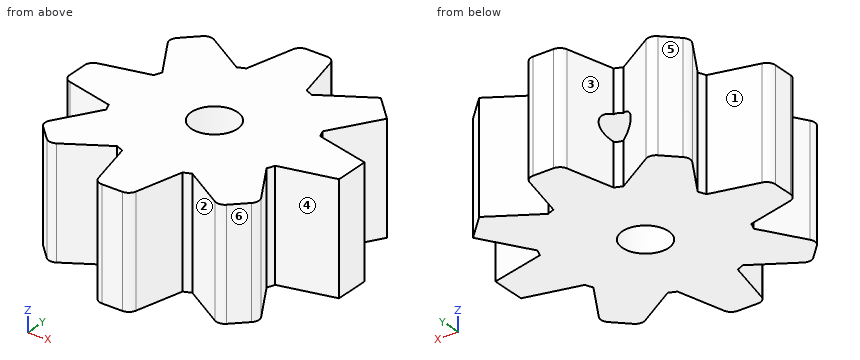
from build123d import *

# Parameters (mm, degrees)
SKETCH1_R                      = 10
SKETCH1_R_2                    = 2.6
BOSS_EXTRUDE1_DEPTH            = 12.4
BOSS_EXTRUDE2_DEPTH            = 6.2
CIRPATTERN1_DEPTH              = 12.4
CUT_EXTRUDE1_REACH             = 35.782
CUT_EXTRUDE1_END_RADIUS        = 2.6
SKETCH5_R                      = 1.5
CUT_EXTRUDE1_DIRECTION_2_DEPTH = 4.1
FILLET4_R                      = 1


# Read off the part's stored shape, not the designer's step: CirPattern1
with BuildPart() as part:
    # Sketch1 → Boss-Extrude1 (new body)
    with BuildSketch(Plane.XY):
        with Locations(Location((0, 0, 0), (0, 0, 180))):
            Circle(SKETCH1_R)
        with Locations(Location((0, 0, 0), (0, 0, 180))):
            Circle(SKETCH1_R_2, mode=Mode.SUBTRACT)
    extrude(amount=BOSS_EXTRUDE1_DEPTH)

    # Sketch2 → Boss-Extrude2 (add, symmetric)
    with BuildSketch(Plane.XY.offset(6.2)):
        Polygon((-1.935099749, 15.52158862), (-3.5, 9), (3.5, 9), (1.935099749, 15.52158862), align=None)
    extrude(amount=BOSS_EXTRUDE2_DEPTH, both=True)

    # CirPattern1 outline → CirPattern1 (add)
    with BuildSketch(Plane.XY):
        with BuildLine():
            Line((-9.607098413, 12.343742723), (-12.343742723, 9.607098413))
            Line((-12.343742723, 9.607098413), (-9.055455951, 4.242489544))
            ThreePointArc((-9.055455951, 4.242489544), (-7.071067812, 7.071067812), (-4.242489544, 9.055455951))
            Line((-4.242489544, 9.055455951), (-9.607098413, 12.343742723))
        make_face()
        with BuildLine():
            ThreePointArc((4.242489544, 9.055455951), (7.071067812, 7.071067812), (9.055455951, 4.242489544))
            Line((9.055455951, 4.242489544), (12.343742723, 9.607098413))
            Line((12.343742723, 9.607098413), (9.607098413, 12.343742723))
            Line((9.607098413, 12.343742723), (4.242489544, 9.055455951))
        make_face()
        with BuildLine():
            ThreePointArc((9.403067435, 3.403281184), (10, 0), (9.403067435, -3.403281184))
            Line((9.403067435, -3.403281184), (15.52158862, -1.935099749))
            Line((15.52158862, -1.935099749), (15.52158862, 1.935099749))
            Line((15.52158862, 1.935099749), (9.403067435, 3.403281184))
        make_face()
        with BuildLine():
            ThreePointArc((9.055455951, -4.242489544), (7.071067812, -7.071067812), (4.242489544, -9.05545595))
            Line((4.242489544, -9.05545595), (9.607098413, -12.343742723))
            Line((9.607098413, -12.343742723), (12.343742723, -9.607098413))
            Line((12.343742723, -9.607098413), (9.055455951, -4.242489544))
        make_face()
        with BuildLine():
            ThreePointArc((3.403281184, -9.403067435), (0, -10), (-3.403281184, -9.403067435))
            Line((-3.403281184, -9.403067435), (-1.935099749, -15.52158862))
            Line((-1.935099749, -15.52158862), (1.935099749, -15.52158862))
            Line((1.935099749, -15.52158862), (3.403281184, -9.403067435))
        make_face()
        with BuildLine():
            ThreePointArc((-4.242489544, -9.05545595), (-7.071067812, -7.071067812), (-9.055455951, -4.242489544))
            Line((-9.055455951, -4.242489544), (-12.343742723, -9.607098413))
            Line((-12.343742723, -9.607098413), (-9.607098413, -12.343742723))
            Line((-9.607098413, -12.343742723), (-4.242489544, -9.05545595))
        make_face()
        with BuildLine():
            ThreePointArc((-9.403067435, -3.403281184), (-10, 0), (-9.403067435, 3.403281184))
            Line((-9.403067435, 3.403281184), (-15.52158862, 1.935099749))
            Line((-15.52158862, 1.935099749), (-15.52158862, -1.935099749))
            Line((-15.52158862, -1.935099749), (-9.403067435, -3.403281184))
        make_face()
    extrude(amount=CIRPATTERN1_DEPTH)

    # Cut-Extrude1: up to this cylinder (the profile starts outside it)
    cut_extrude1_end = Plane(origin=(0, 0, 6.2), z_dir=(0, 0, -1)) * Cylinder(CUT_EXTRUDE1_END_RADIUS, 77.764, mode=Mode.PRIVATE)
    # Sketch5 → Cut-Extrude1 (cut, up to the surface)
    with BuildSketch(Plane(origin=(-3.826834324, 9.238795325, 0), x_dir=(0.9238795325112892, 0.3826834323650838, 0), z_dir=(-0.3826834323650838, 0.9238795325112892, 0)), mode=Mode.PRIVATE) as cut_extrude1_sk1:
        with Locations(Location((0, -6.2, 0), (0, 0, 72.37509472))):
            Circle(SKETCH5_R)
    cut_extrude1_tool1 = extrude(cut_extrude1_sk1.sketch, amount=-CUT_EXTRUDE1_REACH, mode=Mode.PRIVATE) - cut_extrude1_end
    add(cut_extrude1_tool1.solids().sort_by_distance((-3.826834, 9.238795, 6.2))[0], mode=Mode.SUBTRACT)

    # Sketch5 → Cut-Extrude1 direction 2 (cut)
    with BuildSketch(Plane(origin=(-3.826834324, 9.238795325, 0), x_dir=(0.9238795325112892, 0.3826834323650838, 0), z_dir=(-0.3826834323650838, 0.9238795325112892, 0))):
        with Locations(Location((0, -6.2, 0), (0, 0, 72.37509472))):
            Circle(SKETCH5_R)
    extrude(amount=CUT_EXTRUDE1_DIRECTION_2_DEPTH, mode=Mode.SUBTRACT)

    # Fillet4
    fillet4_edges = [part.edges().sort_by_distance(p)[0] for p in [
        (9.607098413, -12.343742723, 6.2),
        (12.343742723, -9.607098413, 6.2),
        (1.935099749, 15.52158862, 6.2),
        (-1.935099749, 15.52158862, 6.2),
        (-9.607098413, 12.343742723, 6.2),
        (-12.343742723, 9.607098413, 6.2),
        (-15.52158862, 1.935099749, 6.2),
        (-15.52158862, -1.935099749, 6.2),
        (-12.343742723, -9.607098413, 6.2),
        (-9.607098413, -12.343742723, 6.2),
        (-1.935099749, -15.52158862, 6.2),
        (1.935099749, -15.52158862, 6.2),
    ]]
    fillet(fillet4_edges, radius=FILLET4_R)


solid = part.part
Geometry: final body of the model. Coordinates: model frame, mm. Face numbers are marked on the shaded views. A direction names the side the tool comes from. Give positions to 0.01 mm unless a question says otherwise; leave off trailing zeros. Write each loop counter-clockwise with the first axis right and the second up, starting at its lowest first coordinate (ties: lowest second). Pieces come first, ordered by that corner, then holes. Notation, with made-up numbers: M 88.25,48 L 117.25,48 A36 cw 117.25,84 Z; hole C -17,89 d6. An arc over 180 degrees is marked long. Answer in a Markdown table with one row per item. Add a question column.
(1) First-contact query: pin 1 (2 mm diameter, centred on y = -9, z = 2, fed in from +X); pin 2 (4 mm diameter, centred on x = 12, y = -5, fed in from -Z); pin 3 (5 mm diameter, centred on x = 6.5, z = 8, fed in from -Y); pin 4 (2 mm diameter, centred on x = -10, z = 6, fed in from +Y). Flat tips, straight axial feed; report the tip coordinate or a pass-through.
(2) Section C-C on y = -8. Return loops of the section in (x, z).
(3) Ray query, line 1 (Y direction, x = 0, z = 2.75); line 2 (X direction, y = -9.5, z = 1.25); line 3 (Y direction, x = 10, z = 10). Return the intervals inside material, ascending.
(4) Reachability of the marked faces 1, 2 and 3 from +Z, -Z, +X, -X, +Y, -Y: full face, straight path, thin tool, end or side. Return the list, or none.
(5) Section A-A on y = 0. Return loops of the section in (x, z), and give its area (3 significant figures).
(6) Mould query, pull axis Y, two halves, no side actions, for the marked faces 4, 5 and 6. Classes: +Y half, -Y half, draft (parallel to the pull), parting line (faces both ways), or undercut.
(7) Section B-B on x = 7.5. Return loops of the section in (y, z), and give its area (3 significant figures).
Result set:
| question | item | result |
|---|---|---|
| 1 | pin 1 | stops at x = 12.08 |
| 1 | pin 2 | passes through |
| 1 | pin 3 | stops at y = -11.97 |
| 1 | pin 4 | stops at y = 12.08 |
| 2 | outline | M -11.36,0 L 11.36,0 L 11.36,12.4 L -11.36,12.4 Z |
| 3 | line 1 | y = -15.52 to -2.6, 2.6 to 15.52 |
| 3 | line 2 | x = -12.08 to -4.97, -3.38 to 3.38, 4.97 to 12.08 |
| 3 | line 3 | y = -11.92 to -5.78, -3.26 to 3.26, 5.78 to 11.95 |
| 4 | face 1 | +Z, -Z, -X |
| 4 | face 2 | +Z, -Z, -Y |
| 4 | face 3 | +Z, -Z, +Y |
| 5 | outline | M -15.52,0 L -2.6,0 L -2.6,12.4 L -15.52,12.4 Z; M 2.6,0 L 15.52,0 L 15.52,12.4 L 2.6,12.4 Z |
| 5 | area | 320 mm^2 |
| 6 | face 4 | undercut |
| 6 | face 5 | +Y half |
| 6 | face 6 | -Y half |
| 7 | outline | M -11.05,0 L 11.05,0 L 11.05,12.4 L -11.05,12.4 Z |
| 7 | area | 274 mm^2 |
